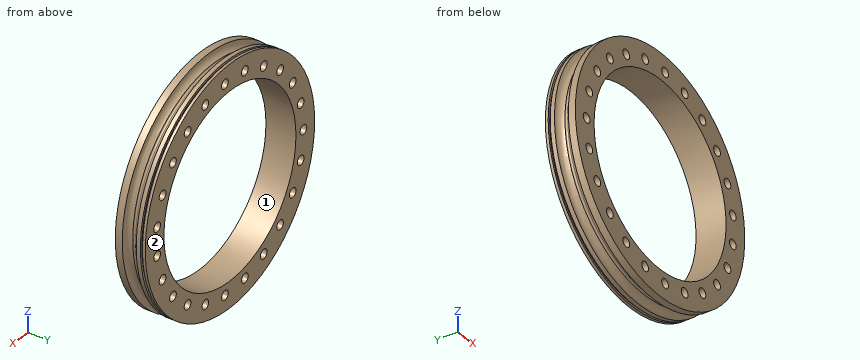
```python
from build123d import *

# Parameters (mm, degrees)
ESQUISSE4_R                  = 6.75
ENL_V_MAT_EXTRU_2_DEPTH      = 245.231447607
R_P_TITION_CIRCULAIRE1_COUNT = 23


with BuildPart() as part:
    # Esquisse1 → R_volution1 (revolve)
    with BuildSketch(Plane.XY):
        with BuildLine():
            Line((-170, 43), (-170, 39))
            Line((-170, 39), (-167, 39))
            Line((-167, 39), (-167, 36))
            Line((-167, 36), (-170, 36))
            Line((-170, 36), (-170, 30))
            ThreePointArc((-170, 30), (-163.666348189, 27.738530528), (-160.197368421, 21.976970948))
            ThreePointArc((-160.197368421, 21.976970948), (-158.5, 20), (-160.197368421, 18.023029052))
            ThreePointArc((-160.197368421, 18.023029052), (-163.666348189, 12.261469472), (-170, 10))
            Line((-170, 10), (-170, 0))
            Line((-170, 0), (-132.5, 0))
            Line((-132.5, 0), (-132.5, 43))
            Line((-132.5, 43), (-170, 43))
        make_face()
    revolve(axis=Axis((0, 43, 0), (0, -1, 0)))

    # Esquisse4 → Enl_v. mat.-Extru.2 (cut, through all)
    with BuildSketch(Plane(origin=(0, 43, 0), x_dir=(1, 0, 0), z_dir=(0, 1, 0))):
        with Locations(Location((-147.5, 0, 0), (0, 0, 270))):
            Circle(ESQUISSE4_R)
    enl_v_mat_extru_2 = extrude(amount=-ENL_V_MAT_EXTRU_2_DEPTH, mode=Mode.SUBTRACT)

    # R_p_tition circulaire1: Enl_v. mat.-Extru.2 ×23 about axis
    r_p_tition_circulaire1_axis = Axis((0, 0, 0), (0, 1, 0))
    for i in range(1, R_P_TITION_CIRCULAIRE1_COUNT):
        add(enl_v_mat_extru_2.rotate(r_p_tition_circulaire1_axis, i * 360 / R_P_TITION_CIRCULAIRE1_COUNT), mode=Mode.SUBTRACT)


solid = part.part
```
The listing builds one solid part. Answer for the finished solid, in the listing's coordinates (mm). Face numbers are marked on the shaded views. Give positions to 0.01 mm unless a question says otherwise; leave off trailing zeros. Loops run counter-clockwise (first coordinate to the right, second up) from the corner with the lowest first, then second, coordinate; pieces in that order, holes last. Notation, with made-up numbers: M 32,39 L 67,39 A34 ccw 67,73 Z; hole C 57,7.25 d11. An arc over 180 degrees is marked long. One line per item, written item: value.
1. For a pull along Z with two mould halves and no side action, classify the marked faces 1 and 2 as pulls with the +Z half, pulls with the -Z half, needs draft (parallel to the pull), parting line crosses it, or undercut.
Found:
face 1: undercut
face 2: needs draft
2. Section A-A on z = 0 is taken. Determine the outline of the cut face in (x, y).
Found:
outline: M -170,0 L -154.25,0 L -154.25,43 L -170,43 L -170,39 L -167,39 L -167,36 L -170,36 L -170,30 A10 cw -160.2,21.98 A2 cw -160.2,18.02 A10 cw -170,10 Z; M -140.75,0 L -132.5,0 L -132.5,43 L -140.75,43 Z; M 132.5,0 L 170,0 L 170,10 A10 cw 160.2,18.02 A2 cw 160.2,21.98 A10 cw 170,30 L 170,36 L 167,36 L 167,39 L 170,39 L 170,43 L 132.5,43 Z
3. Each of these flat-tipped pins is pushed along its axis until it touches: P1, Ø12, axis at x = -30.01, z = 144.41, coming from the -Y side; P2, Ø1.5, axis at x = 69.5, y = 13.5, coming from the +Z side; P3, Ø4, axis at x = 23.5, y = 33, coming from the -Z side; P4, Ø12, axis at x = 37, y = 8, coming from the +Z side. Where does it stop, or does it pass through?
Found:
P1: through
P2: z = 147.63
P3: z = -168.63
P4: z = 167.15
4. Section B-B on y = 4 is taken. State how many separate pieces and enclosed holes the cut face has, plus the area to 3 significant figures.
Found:
separate pieces: 1
enclosed holes: 24
area: 32,300 mm^2
5. Find the intervals of material crossed by probe 1 along Z at (x, y) = (82, 13); probe 2 along X at (y, z) = (28, 107); probe 3 along X at (y, z) = (38, 14), in increasing order.
Found:
probe 1: -140.71 to -126.52, -114.49 to -104.08, 104.08 to 114.49, 126.52 to 140.71
probe 2: -124.29 to -107.38, -93.97 to -78.15, 78.15 to 124.29
probe 3: -166.41 to -131.76, 131.76 to 143.2, 149.05 to 166.41
